Part print with two shaded views. Sizes in mm from the minimum x, y, z corner. A direction names the side the tool comes from. Give positions to 0.01 mm unless a question says otherwise; leave off trailing zeros. Write each loop counter-clockwise with the first axis right and the second up, starting at its lowest first coordinate (ties: lowest second). Pieces come first, ordered by that corner, then holes.
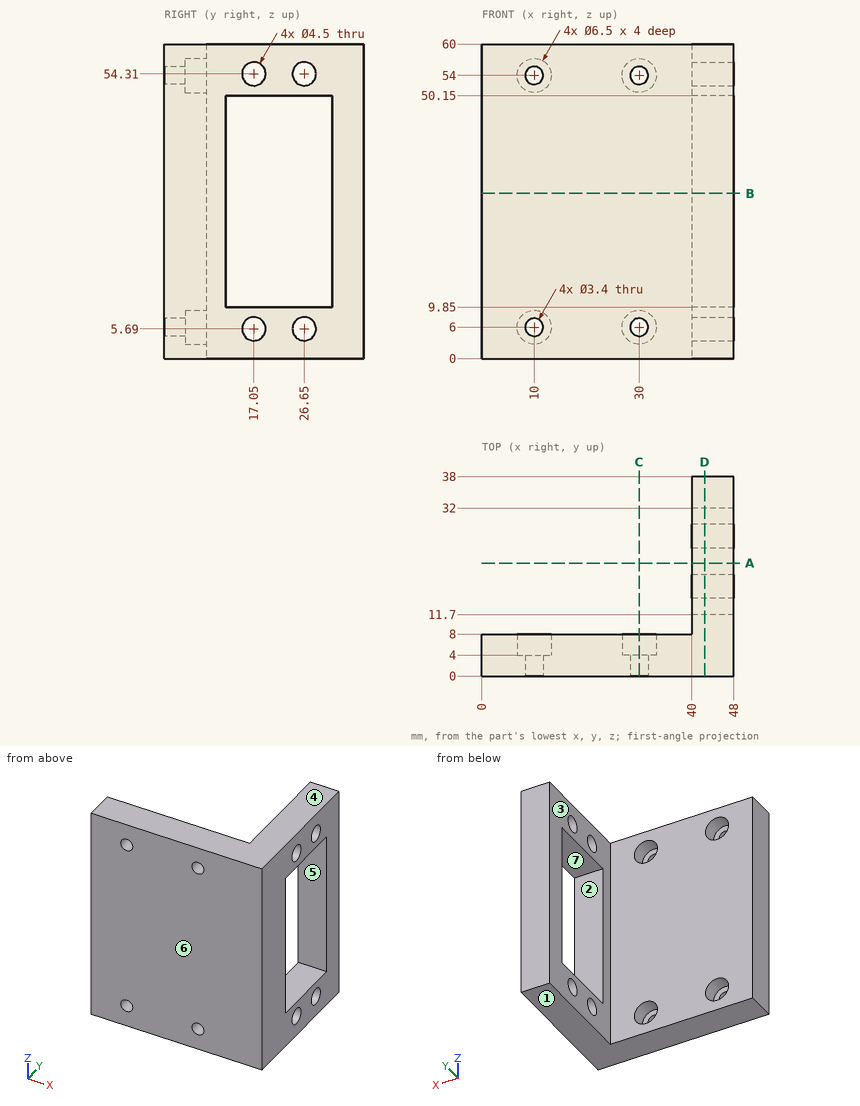
1) Saw through at A-A (y = 21.5). Write the cut outline in (x, z), and give its area (3 significant figures).
Check result:
outline: (40, 0) - (48, 0) - (48, 9.85) - (40, 9.85) - close; (40, 50.15) - (48, 50.15) - (48, 60) - (40, 60) - close
area: 158 mm2
2) Drill centre lines: L1, parallel to Y at x = 46.25, z = 54.31; L2, parallel to Z at x = 44, y = 17; L3, parallel to Z at x = 30, y = 1.5. Where is each one in solid material? Low to high.
Check result:
L1: y = 0 to 14.8, 19.3 to 24.4, 28.9 to 38
L2: z = 0 to 3.44, 7.94 to 9.85, 50.15 to 52.06, 56.56 to 60
L3: z = 0 to 4.3, 7.7 to 52.3, 55.7 to 60
3) 3-axis set-ups, long thin cutter, end or side, ignore diameter. For the marked faces 1, 2 and 3: which of +Z, -Z, +X, -X, +Y, -Y reach the whole face in a straight line?
Check result:
face 1: -Z, +X, -X, +Y, -Y
face 2: +X, -X
face 3: +Z, -Z, -X, +Y
4) Saw through at D-D (x = 42.5). Write the cut outline in (y, z).
Check result:
outline: (0, 0) - (38, 0) - (38, 60) - (0, 60) - close; hole (11.7, 9.85) - (32, 9.85) - (32, 50.15) - (11.7, 50.15) - close; hole circle Ø4.5 at (17.05, 5.69); hole circle Ø4.5 at (17.05, 54.31); hole circle Ø4.5 at (26.65, 5.69); hole circle Ø4.5 at (26.65, 54.31)
5) Saw through at C-C (x = 30). Write the cut outline in (y, z).
Check result:
outline: (0, 0) - (8, 0) - (8, 2.75) - (4, 2.75) - (4, 4.3) - (0, 4.3) - close; (0, 7.7) - (4, 7.7) - (4, 9.25) - (8, 9.25) - (8, 50.75) - (4, 50.75) - (4, 52.3) - (0, 52.3) - close; (0, 55.7) - (4, 55.7) - (4, 57.25) - (8, 57.25) - (8, 60) - (0, 60) - close
6) Saw through at B-B (z = 31.5). Write the cut outline in (x, y), and give its area (3 significant figures).
Check result:
outline: (0, 0) - (48, 0) - (48, 11.7) - (40, 11.7) - (40, 8) - (0, 8) - close; (40, 32) - (48, 32) - (48, 38) - (40, 38) - close
area: 462 mm2
7) Flat gauge pins, fed straight in: P1, Ø3, axis at x = 9.5, z = 53, coming from the +Y side; P2, Ø5, axis at y = 26.65, z = 5.69, coming from the -X side; P3, Ø7, axis at x = 31, z = 52.5, coming from the +Y side. Where does each tip first touch, or does it go through?
Check result:
P1: stops at y = 4
P2: stops at x = 40
P3: stops at y = 8
8) Mould opens along Z. For the marked faces 4, 5, 6 and 7 say: +Z half, -Z half, draft (parallel to the pull), parting line (faces both ways), or undercut.
Check result:
face 4: +Z half
face 5: undercut
face 6: draft
face 7: undercut
